Read the model definition and answer for the solid it produces. Units are mm, in the model's axes. Coordinates: 2 decimals unless noted, no trailing zeros. Write item = value, one per line.
from build123d import *

# Parameters (mm, degrees)
CUT_EXTRUDE_START         = -16.803249302
CUT_EXTRUDE_1_OUTLINE_R   = 1
CUT_EXTRUDE_1_OUTLINE_R_2 = 12.5
CUT_EXTRUDE_1_OUTLINE_R_3 = 10.000000001
CUT_EXTRUDE_1_DEPTH       = 16.803249302
FILLET_1_R                = 2


# Read off the part's stored shape, not the designer's step: the extrude step
with BuildPart() as part:
    # Sketch 1 → Revolve 1 (revolve)
    with BuildSketch(Plane(origin=(0, 0, 0), x_dir=(1, 0, 0), z_dir=(0, 1, 0)), mode=Mode.PRIVATE) as revolve_1_sk:
        with BuildLine():
            add(Edge.make_bspline(
                [(17.433204834, 10.06506551), (17.337637394, 10.327692888), (17.033613112, 11.118040994), (16.453706626, 12.40909657), (15.480365784, 14.138500707), (14.153596875, 15.999234034), (12.853752585, 17.466352611), (11.847269766, 18.426266867), (11.224854433, 18.96410642), (11.038988479, 19.120088927)],
                knots=[0.032150936, 0.032150936, 0.032150936, 0.032150936, 0.032150936, 0.03330181, 0.035637492, 0.037972373, 0.040307253, 0.042695151, 0.043694361, 0.043694361, 0.043694361, 0.043694361, 0.043694361], degree=4))
            Line((17.433204862, 10.06506552), (26.42596579, 15.257038463))
            Line((26.42596579, 15.257038463), (21.242021226, 22.598163159))
            Line((21.242021226, 22.598163159), (16.733350813, 28.983013789))
            Line((16.733350813, 28.983013789), (11.038988511, 19.120088966))
        make_face()
        with BuildLine():
            Line((11.038988511, 19.120088966), (17.433204862, 10.06506552))
            add(Edge.make_bspline(
                [(17.433204834, 10.06506551), (17.337637394, 10.327692888), (17.033613112, 11.118040994), (16.453706626, 12.40909657), (15.480365784, 14.138500707), (14.153596875, 15.999234034), (12.853752585, 17.466352611), (11.847269766, 18.426266867), (11.224854433, 18.96410642), (11.038988479, 19.120088927)],
                knots=[0.032150936, 0.032150936, 0.032150936, 0.032150936, 0.032150936, 0.03330181, 0.035637492, 0.037972373, 0.040307253, 0.042695151, 0.043694361, 0.043694361, 0.043694361, 0.043694361, 0.043694361], degree=4))
        make_face()
    revolve(revolve_1_sk.sketch.rotate(Axis((35.122395357, 0, -20.277924414), (-0.576829805989874, 0, -0.8168643552767402)), 180), axis=Axis((35.122395357, 0, -20.277924414), (-0.576829805989874, 0, -0.8168643552767402)))

    # Cut-Extrude 1 outline → Cut-Extrude 1 (cut)
    # profile 1 of 7: a face of its own
    with BuildSketch(Plane(origin=(1.603790962, 0, 2.271171941), x_dir=(0.8168643552767402, 0, -0.576829805989874), z_dir=(0.576829805989874, 0, 0.8168643552767403)).offset(CUT_EXTRUDE_START)):
        with BuildLine():
            ThreePointArc((30.654467809, 17.861163132), (22.771537413, 10.170375515), (20.052584902, -0.501836207))
            ThreePointArc((20.052584902, -0.501836207), (27.396763211, 7.500000385), (30.654467809, 17.861163132))
        make_face()
    # profile 2 of 7: a face of its own
    with BuildSketch(Plane(origin=(1.603790962, 0, 2.271171941), x_dir=(0.8168643552767402, 0, -0.576829805989874), z_dir=(0.576829805989874, 0, 0.8168643552767403)).offset(CUT_EXTRUDE_START)):
        with BuildLine():
            ThreePointArc((50.989026765, -17.359326803), (40.387143684, -15), (29.785260672, -17.359327109))
            ThreePointArc((29.785260672, -17.359327109), (40.387143846, -20.340750604), (50.989026765, -17.359326803))
        make_face()
    # profile 3 of 7: a face of its own
    with BuildSketch(Plane(origin=(1.603790962, 0, 2.271171941), x_dir=(0.8168643552767402, 0, -0.576829805989874), z_dir=(0.576829805989874, 0, 0.8168643552767403)).offset(CUT_EXTRUDE_START)):
        with BuildLine():
            ThreePointArc((60.721703188, -0.501836207), (58.002750779, 10.170375338), (50.11982064, 17.861162936))
            ThreePointArc((50.11982064, 17.861162936), (53.377525064, 7.500000066), (60.721703188, -0.501836207))
        make_face()
    # profile 4 of 7: a face of its own
    with BuildSketch(Plane(origin=(1.603790962, 0, 2.271171941), x_dir=(0.8168643552767402, 0, -0.576829805989874), z_dir=(0.576829805989874, 0, 0.8168643552767403)).offset(CUT_EXTRUDE_START)):
        with Locations((55.837687291, -8.920375302)):
            Circle(CUT_EXTRUDE_1_OUTLINE_R)
    # profile 5 of 7: a face of its own
    with BuildSketch(Plane(origin=(1.603790962, 0, 2.271171941), x_dir=(0.8168643552767402, 0, -0.576829805989874), z_dir=(0.576829805989874, 0, 0.8168643552767403)).offset(CUT_EXTRUDE_START)):
        with Locations((40.387144045, 0)):
            Circle(CUT_EXTRUDE_1_OUTLINE_R_2)
        with Locations((40.387144045, 0)):
            Circle(CUT_EXTRUDE_1_OUTLINE_R_3, mode=Mode.SUBTRACT)
    # profile 6 of 7: a face of its own
    with BuildSketch(Plane(origin=(1.603790962, 0, 2.271171941), x_dir=(0.8168643552767402, 0, -0.576829805989874), z_dir=(0.576829805989874, 0, 0.8168643552767403)).offset(CUT_EXTRUDE_START)):
        with Locations((40.387144045, 17.840750604)):
            Circle(CUT_EXTRUDE_1_OUTLINE_R)
    # profile 7 of 7: a face of its own
    with BuildSketch(Plane(origin=(1.603790962, 0, 2.271171941), x_dir=(0.8168643552767402, 0, -0.576829805989874), z_dir=(0.576829805989874, 0, 0.8168643552767403)).offset(CUT_EXTRUDE_START)):
        with Locations((24.9366008, -8.920375302)):
            Circle(CUT_EXTRUDE_1_OUTLINE_R)
    extrude(amount=CUT_EXTRUDE_1_DEPTH, mode=Mode.SUBTRACT)

    # Fillet 1
    fillet_1_edges = [part.edges().sort_by_distance(p)[0] for p in [
        (24.251858401, 2e-09, -14.001816977),
    ]]
    fillet(fillet_1_edges, radius=FILLET_1_R)


solid = part.part
1) Straight lines are drawn through the part: line 1 along Y through (x, z) = (19.5, -23.5); line 2 along Y through (x, z) = (30, -32); line 3 along X through (y, z) = (-2, -11.5). For each, find the intervals that lie inside material, in ascending order. Write a range as from..to.
Returned:
line_1 = -17.17..-6.11, 6.11..12.16
line_2 = -15.13..-12.23, 12.23..20.18
line_3 = 16.54..19.9
2) Determine the mould class of faces 1 (the face through (30, -15, -27)), 2 (the face through (16.6, -10.3, -16.1)), 3 (the face through (40.774, 7.633, -34.662)) for opening direction Z: pulls with the +Z half, pulls with the -Z half, needs draft (parallel to the pull), parting line crosses it, or undercut.
Returned:
face_1 = undercut
face_2 = pulls with the +Z half
face_3 = pulls with the -Z half
3) The part is cut by section A-A (x = 29). Count the separate pieces of the cut face and the enclosed holes in it, and give its area (3 significant figures).
Returned:
separate_pieces = 2
enclosed_holes = 1
area = 178 mm^2
4) Flat-ended cylindrical pins translate along their axes: pin 1 Ø3 at (x, z) = (31.5, -32) entering from -Y; pin 2 Ø4 at (y, z) = (5, -14) entering from +X; pin 3 Ø12 at (x, z) = (34, -22) entering from -Y. Find the tip coordinate at first contact, or state that the pin passes through.
Returned:
pin_1 = -15.57
pin_2 = 24.75
pin_3 = -15.75
